```python
from build123d import *

# Parameters (mm, degrees)
CROQUIS1_W              = 25.4
CROQUIS1_H              = 25.4
CROQUIS1_W_2            = 21.4
CROQUIS1_H_2            = 21.4
SALIENTE_EXTRUIR1_DEPTH = 1150
REDONDEO1_R             = 2
CROQUIS2_R              = 2.5
CORTAR_EXTRUIR1_DEPTH   = 10
MATRIZL1_COUNT          = 4
MATRIZL1_PITCH          = 357.9333
CROQUIS3_R              = 6
CORTAR_EXTRUIR2_DEPTH   = 10
MATRIZL2_COUNT          = 4
MATRIZL2_PITCH          = 357.9333


with BuildPart() as part:
    # Croquis1 → Saliente-Extruir1 (new body)
    with BuildSketch(Plane.XY):
        Rectangle(CROQUIS1_W, CROQUIS1_H)
        Rectangle(CROQUIS1_W_2, CROQUIS1_H_2, mode=Mode.SUBTRACT)
    extrude(amount=SALIENTE_EXTRUIR1_DEPTH)

    # Redondeo1
    redondeo1_edges = [part.edges().sort_by_distance(p)[0] for p in [
        (-10.7, 10.7, 575),
        (-10.7, -10.7, 575),
        (10.7, -10.7, 575),
        (10.7, 10.7, 575),
        (-12.7, 12.7, 575),
        (12.7, 12.7, 575),
        (12.7, -12.7, 575),
        (-12.7, -12.7, 575),
    ]]
    fillet(redondeo1_edges, radius=REDONDEO1_R)

    # Croquis2 → Cortar-Extruir1 (cut)
    with BuildSketch(Plane(origin=(0, 12.7, 0), x_dir=(1, 0, 0), z_dir=(0, 1, 0))):
        with Locations(Location((0, -1111.9, 0), (0, 0, 180))):
            Circle(CROQUIS2_R)
    cortar_extruir1 = extrude(amount=-CORTAR_EXTRUIR1_DEPTH, mode=Mode.SUBTRACT)

    # MatrizL1: Cortar-Extruir1 ×4
    with Locations(*[(0, 0, -i * MATRIZL1_PITCH) for i in range(1, MATRIZL1_COUNT)]):
        add(cortar_extruir1, mode=Mode.SUBTRACT)

    # Croquis3 → Cortar-Extruir2 (cut)
    with BuildSketch(Plane.XZ.offset(12.7)):
        with Locations((0, 1111.9)):
            Circle(CROQUIS3_R)
    cortar_extruir2 = extrude(amount=-CORTAR_EXTRUIR2_DEPTH, mode=Mode.SUBTRACT)

    # MatrizL2: Cortar-Extruir2 ×4
    with Locations(*[(0, 0, -i * MATRIZL2_PITCH) for i in range(1, MATRIZL2_COUNT)]):
        add(cortar_extruir2, mode=Mode.SUBTRACT)


solid = part.part
```
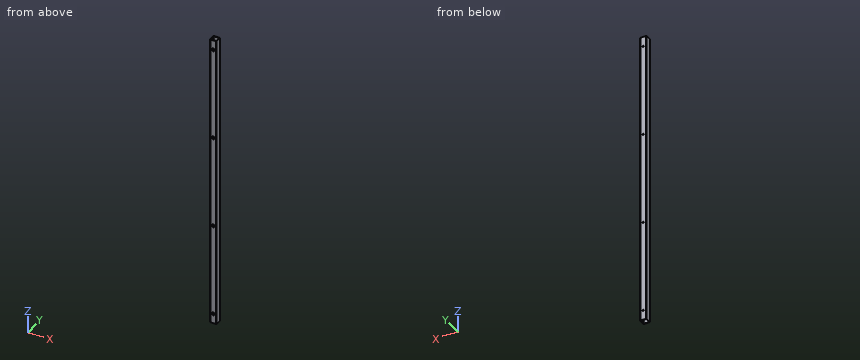
Geometry: final body of the model. Coordinates: model frame, mm. Coordinates: 2 decimals unless noted, no trailing zeros. Write each loop counter-clockwise with the first axis right and the second up, starting at its lowest first coordinate (ties: lowest second). Pieces come first, ordered by that corner, then holes. Notation, with made-up numbers: M 45.25,19 L 50.25,19 A27 ccw 50.25,42 Z; hole C 79.25,75.25 d2. An arc over 180 degrees is marked long. Answer as CSV lines item,"result". Start each with the question number.
Q1. Cut plane A-A on y = 0. Return the cut outline in (x, z).
Q2. Cut plane B-B on z = 942.5. Return the cut outline in (x, y), then the cut area to 3 significant figures.
Q3. Line query: line 1 (Z direction, x = 0, y = 11.6); line 2 (Z direction, x = 0, y = -11.8); line 3 (Y direction, x = -7, z = 435). Output: solid intervals per line, ascending. Write a range as from..to.
Q4. Pin query (flat end, axial travel): P1, Ø1.5, axis at x = -8.5, y = -7, coming from the +Z side; P2, Ø6.5, axis at x = 0, z = 753.97, coming from the -Y side. Return the tip coordinate at first contact, or that it passes through.
Findings below:
1,outline,"M -12.7,0 L -10.7,0 L -10.7,1150 L -12.7,1150 Z; M 10.7,0 L 12.7,0 L 12.7,1150 L 10.7,1150 Z"
2,outline,"M -12.7,-10.7 A2 ccw -10.7,-12.7 L 10.7,-12.7 A2 ccw 12.7,-10.7 L 12.7,10.7 A2 ccw 10.7,12.7 L -10.7,12.7 A2 ccw -12.7,10.7 Z; hole M -10.7,-8.7 A2 ccw -8.7,-10.7 L 8.7,-10.7 A2 ccw 10.7,-8.7 L 10.7,8.7 A2 ccw 8.7,10.7 L -8.7,10.7 A2 ccw -10.7,8.7 Z"
2,area,"187 mm2"
3,line 1,"z = 0..35.6, 40.6..393.53, 398.53..751.47, 756.47..1109.4, 1114.4..1150"
3,line 2,"z = 0..32.1, 44.1..390.03, 402.03..747.97, 759.97..1105.9, 1117.9..1150"
3,line 3,"y = -12.7..-10.7, 10.7..12.7"
4,P1,"passes through"
4,P2,"stops at y = 10.7"
